Here's how the part is built. I have some questions about the finished solid (model axes, mm). A direction names the side the tool comes from. Coordinates: 2 decimals unless noted, no trailing zeros. Write each loop counter-clockwise with the first axis right and the second up, starting at its lowest first coordinate (ties: lowest second). Pieces come first, ordered by that corner, then holes. Notation, with made-up numbers: (-9.5, 48.25) -> (16.5, 48.25) arc R36 ccw to (16.5, 87.25) -> close; hole circle Ø9 at (64, -35.75). An arc over 180 degrees is marked (long way). Put each result on its own line as item: value. Start each with the question number.
Item 1: If we mould it in two halves opening along X, with no side actions, what happens to faces 1 (the face through (99.512, -2.276, 6.282)), 2 (the face through (-100.488, -2.276, 6.282)), 3 (the face through (140, -4, 8)), 4 (the face through (-140, -4, 8))? For each: released by +X, released by -X, zero draft, split by the parting line, or undercut.
Item 2: I want a section at A-A, the plane z = 10. List the corners of the cut face in (x, y) for me, then the cut area to 3 significant figures.
Item 3: I need wall thicknesses on line 1 (X direction, y = -0.5, z = 10); line 2 (Z direction, x = 100, y = -8.85); line 3 (X direction, y = -2.75, z = 8.5). Which ranges of each line are inside material? Lowest first, please. Write a range as [from, to].
Item 4: On a 3-axis mill with a long thin cutter (end or side, diameter ignored), from which of +Z, -Z, +X, -X, +Y, -Y can I reach the whole of each face in a straight line? I mean faces 5 (the face through (102, -5, 12)), 6 (the face through (-2, -7, 20)). Say none if no direction works.
Item 5: For pin 1 (4 mm diameter, centred on x = -101, z = 10.5, fed in from +Y); pin 2 (1 mm diameter, centred on x = 0.5, z = 17, fed in from +Y); pin 3 (4 mm diameter, centred on x = 13.5, z = 18, fed in from +Y); pin 4 (4 mm diameter, centred on x = -100, z = 10, fed in from +Y), each with a flat end and sliding along its axis, tell me the tip position at first contact or that it passes through.
Item 6: I want a section at C-C, the plane y = -2.25. List the corners of the cut face in (x, z) for me, then the cut area to 3 significant figures.
Item 7: I want a section at B-B, the plane x = -100. List the corners of the cut face in (y, z) for me (3 decimals), then the cut area to 3 significant figures.
Autodesk Inventor part; units mm, degrees
ref_plane "YZ Plane" through (0, 0, 0) normal (1, 0, 0) x (0, 1, 0)
ref_plane "XZ Plane" through (0, 0, 0) normal (0, 1, 0) x (-1, 0, 0)
ref_plane "XY Plane" through (0, 0, 0) normal (0, 0, 1) x (1, 0, 0)
sketch "Sketch1" plane through (0, 0, 0) normal (0, 0, 1) x (1, 0, 0)
  line L0 (140, 5) -> (-140, 5)
  line L1 (-140, 5) -> (-140, -5)
  line L2 (-140, -5) -> (140, -5)
  line L3 (140, -5) -> (140, 5)
  line L4 (140, 5) -> (-140, -5) construction
  line L5 (-140, 5) -> (140, -5) construction
  point P0 (0, 0)
  dimension "d0" = 280
  dimension "d1" = 10
extrude "Extrusion1" add sketch "Sketch1" along normal blind 20
sketch "Sketch6" plane through (-140, -5, 0) normal (0, -1, 0) x (1, 0, 0)
  line L0 (0, 0) -> (0, 20)
  line L1 (0, 0) -> (280, 0)
  line L2 (0, 20) -> (280, 20)
  line L3 (280, 20) -> (280, 0)
  line L4 (280, 0) -> (0, 0)
  line L5 (0, 0) -> (0, 20)
  point P0 (140, 0)
extrude "Extrusion4" add sketch "Sketch6" along normal blind 5
sketch "Sketch7" plane through (-140, -10, 0) normal (0, -1, 0) x (1, 0, 0)
  point P0 (140, 0)
sketch "Sketch8" plane through (-140, -10, 0) normal (0, -1, 0) x (1, 0, 0)
  circle A0 centre (40, 10) radius 2.1
  circle A1 centre (40, 10) radius 2.25
  circle A2 centre (240, 10) radius 2.25
  line L0 (280, 20) -> (0, 20)
  line L1 (0, 20) -> (0, 0)
  point P0 (140, 0)
  dimension "d23" = 4.5
  dimension "d24" = 4.5
  dimension "d35" = 200
  dimension "d36" = 10
  dimension "d37" = 10
  dimension "d38" = 40
extrude "Extrusion5" cut sketch "Sketch8" against normal through all contours A0 | A1 | A2
sketch "Sketch9" plane through (-140, 5, 0) normal (0, 1, 0) x (1, 0, 0)
  circle A0 centre (40, -10) radius 2.25
  circle A1 centre (40, -10) radius 3.75
  circle A2 centre (240, -10) radius 2.25
  circle A3 centre (240, -10) radius 3.75
  point P0 (140, 0)
  dimension "d27" = 7.5
  dimension "d28" = 7.5
extrude "Extrusion6" cut sketch "Sketch9" against normal blind 10 contours A0 | A1 | A2 | A3
sketch "Sketch10" plane through (-140, 5, 0) normal (-1, 0, 0) x (0, 0, 1)
  line L0 (0, 0) -> (20, 0)
  line L1 (20, 0) -> (20, -10)
  line L2 (20, 0) -> (20, -15)
  line L3 (20, 0) -> (30, 0) construction
  line L4 (0, 0) -> (0, -15)
  line L5 (20, -10) -> (0, 0)
  line L6 (0, 0) -> (20, 0)
  point P0 (0, -5)
  dimension "d31" = 10
  dimension "d32" = 90
extrude "Extrusion7" cut sketch "Sketch10" against normal through all
equation "\"d24\" = d23"
equation "\"d28\" = d27"
properties part number "paw shelf_v03_temp"
Calculated:
1. face 1: undercut
1. face 2: undercut
1. face 3: released by +X
1. face 4: released by -X
2. outline: (-140, -10) -> (-102.25, -10) -> (-102.25, -5) -> (-103.75, -5) -> (-103.75, 0) -> (-140, 0) -> close; (-97.75, -10) -> (97.75, -10) -> (97.75, -5) -> (96.25, -5) -> (96.25, 0) -> (-96.25, 0) -> (-96.25, -5) -> (-97.75, -5) -> close; (102.25, -10) -> (140, -10) -> (140, 0) -> (103.75, 0) -> (103.75, -5) -> (102.25, -5) -> close
2. area: 2,680 mm2
3. line 1: x = [-140, -103.75], [-96.25, 96.25], [103.75, 140]
3. line 2: z = [0, 7.75], [12.25, 20]
3. line 3: x = [-140, -103.44], [-96.56, 96.56], [103.44, 140]
4. face 5: +Y
4. face 6: +Z, +X, -X, +Y, -Y
5. pin 1: stops at y = -5
5. pin 2: stops at y = -3.25
5. pin 3: stops at y = -3
5. pin 4: passes through
6. outline: (-140, 0) -> (140, 0) -> (140, 14.5) -> (-140, 14.5) -> close; hole circle Ø7.5 at (-100, 10); hole circle Ø7.5 at (100, 10)
6. area: 3,970 mm2
7. outline: (-10, 0) -> (5, 0) -> (1.875, 6.25) -> (-5, 6.25) -> (-5, 7.75) -> (-10, 7.75) -> close; (-10, 12.25) -> (-5, 12.25) -> (-5, 13.75) -> (-1.875, 13.75) -> (-5, 20) -> (-10, 20) -> close
7. area: 140 mm2
